Design review of the part built by this model. Coordinates are the model's own, in mm. A direction names the side the tool comes from. Give positions to 0.01 mm unless a question says otherwise; leave off trailing zeros. Loops run counter-clockwise (first coordinate to the right, second up) from the corner with the lowest first, then second, coordinate; pieces in that order, holes last. Notation, with made-up numbers: (28.5, 10.5) -> (36.5, 10.5) arc R23 cw to (36.5, 29.5) -> close; hole circle Ø9 at (-14.5, 49.25). An arc over 180 degrees is marked (long way). Answer as CSV lines item,"result".
from build123d import *

# Parameters (mm, degrees)
BOSS_EXTRUDE1_DEPTH              = 8
CLAMPMOUNTHOLESKETCH2_R          = 2
CLAMPMOUNTHOLECUT_EXTRUDE1_DEPTH = 4.1


with BuildPart() as part:
    # Sketch1 → Boss-Extrude1 (new body)
    with BuildSketch(Plane(origin=(0, 0, 0), x_dir=(0, 0, -1), z_dir=(1, 0, 0))):
        with BuildLine():
            Line((0, 1.381049961), (0, -9.618950039))
            Line((0, -9.618950039), (-4.2, -9.618950039))
            Line((-4.2, -9.618950039), (-4.2, -1.618950039))
            ThreePointArc((-4.2, -1.618950039), (-10.64, 4.821049961), (-4.2, 11.261049961))
            Line((-4.2, 11.261049961), (0, 11.261049961))
            Line((0, 11.261049961), (0, 8.261049961))
            Line((0, 8.261049961), (-4.2, 8.261049961))
            ThreePointArc((-4.2, 8.261049961), (-7.64, 4.821049961), (-4.2, 1.381049961))
            Line((-4.2, 1.381049961), (0, 1.381049961))
        make_face()
    extrude(amount=BOSS_EXTRUDE1_DEPTH)

    # ClampMountHoleSketch2 → ClampMountHoleCut-Extrude1 (cut)
    with BuildSketch(Plane(origin=(0, 0, 0), x_dir=(-1, 0, 0), z_dir=(0, 0, -1))):
        with Locations(Location((-4, -5.618950039, 0), (0, 0, 90))):
            Circle(CLAMPMOUNTHOLESKETCH2_R)
    extrude(amount=-CLAMPMOUNTHOLECUT_EXTRUDE1_DEPTH, mode=Mode.SUBTRACT)


solid = part.part
Q1. We need section B-B, the plane x = 6.75. State the section outline as (y, z) points, and give its area (3 significant figures).
Filled sheet:
outline,"(-9.62, 0) -> (1.38, 0) -> (1.38, 4.2) arc R3.44 cw to (8.26, 4.2) -> (8.26, 0) -> (11.26, 0) -> (11.26, 4.2) arc R6.44 ccw to (-1.62, 4.2) -> (-9.62, 4.2) -> close"
area,"105 mm^2"
Q2. We need section C-C, the plane z = 6. State the section outline as (x, y) points, and give its area (3 significant figures).
Filled sheet:
outline,"(0, -1.36) -> (8, -1.36) -> (8, 1.89) -> (0, 1.89) -> close; (0, 7.75) -> (8, 7.75) -> (8, 11) -> (0, 11) -> close"
area,"52.0 mm^2"
Q3. To check wall thickness, follow probe 1 along Y at (x, z) = (7, 2.75); probe 2 along Y at (x, z) = (6.25, 4.25); probe 3 along Z at (x, y) = (0.5, -2.5). State the ranges of each line that lie inside material, in increasing order. Write a range as from..to.
Filled sheet:
probe 1,"y = -9.62..1.38, 8.26..11.26"
probe 2,"y = -1.62..1.38, 8.26..11.26"
probe 3,"z = 0..4.2"
Q4. The part is to be moulded in two halves that separate along Y. For faces 3 (the cylindrical face through (2.783, -7.206, 2.021)), 4 (the flat face through (4, -9.619, 2)), 5 (the flat face through (0, 1, 4)), 6 (the cylindrical face through (3.94, 4.9, 7.64)), say which applies: pulls with the +Y half, pulls with the -Y half, needs draft (parallel to the pull), parting line crosses it, or undercut.
Filled sheet:
face 3,"undercut"
face 4,"pulls with the -Y half"
face 5,"needs draft"
face 6,"undercut"
Q5. For faces 1 (the flat face through (4, -3, 0)), 2 (the flat face through (4, 1.381, 2)), list the 3-axis set-ups (+Z, -Z, +X, -X, +Y, -Y) from which the entire face can be reached by the end or side of a thin tool; tool diameter is ignored.
Filled sheet:
face 1,"-Z, +X, -X, +Y, -Y"
face 2,"-Z, +X, -X"
Q6. We need section A-A, the plane z = 1.75. State the section outline as (x, y) points, and give its area (3 significant figures).
Filled sheet:
outline,"(0, -9.62) -> (8, -9.62) -> (8, 1.38) -> (0, 1.38) -> close; (0, 8.26) -> (8, 8.26) -> (8, 11.26) -> (0, 11.26) -> close; hole circle Ø4 at (4, -5.62)"
area,"99.4 mm^2"
Q7. We need section D-D, the plane y = -7.25. State the section outline as (x, z) points.
Filled sheet:
outline,"(0, 0) -> (2.84, 0) -> (2.84, 4.1) -> (5.16, 4.1) -> (5.16, 0) -> (8, 0) -> (8, 4.2) -> (0, 4.2) -> close"
Q8. Clearance check with flat-ended pins moving along their axes: pin 1 Ø2.5 at (x, y) = (4, -5) entering from +Z; pin 2 Ø1.5 at (x, y) = (6.5, 1) entering from +Z. State where each tip first meets the part, or that it passes through.
Filled sheet:
pin 1,"stops at z = 4.2"
pin 2,"stops at z = 9.86"
